```python
from build123d import *

# Parameters (mm, degrees)
SKETCH3_W               = 120
SKETCH3_H               = 85
BOSS_EXTRUDE1_DEPTH     = 5
SKETCH4_W               = 45
SKETCH4_H               = 18.75
BOSS_EXTRUDE2_DEPTH     = 20
SKETCH6_W               = 45
SKETCH6_H               = 2
BOSS_EXTRUDE3_DEPTH     = 40
CUT_EXTRUDE1_DEPTH      = 87.204698248
CUT_EXTRUDE1_DEPTH_BACK = 20
SKETCH7_W               = 4
SKETCH7_H               = 2
SKETCH8_W               = 10
SKETCH8_H               = 20
BOSS_EXTRUDE4_DEPTH     = 9
BOSS_EXTRUDE5_DEPTH     = 5.5
SKETCH10_W              = 2
SKETCH10_H              = 5.5
CUT_EXTRUDE2_DEPTH      = 91.627068942
SKETCH11_W              = 10
SKETCH11_H              = 10
BOSS_EXTRUDE6_DEPTH     = 2
SKETCH12_W              = 10
SKETCH12_H              = 10
BOSS_EXTRUDE7_DEPTH     = 9
SKETCH13_W              = 2.4
SKETCH13_H              = 10
BOSS_EXTRUDE8_DEPTH     = 4.5
SKETCH14_W              = 10
SKETCH14_H              = 5
BOSS_EXTRUDE9_DEPTH     = 2
SKETCH15_R              = 1.3
BOSS_EXTRUDE10_DEPTH    = 8
SKETCH16_W              = 9
SKETCH16_H              = 1.5
BOSS_EXTRUDE11_DEPTH    = 8
SKETCH18_W              = 120
SKETCH18_H              = 5
BOSS_EXTRUDE12_DEPTH    = 5
SKETCH19_W              = 90
SKETCH19_H              = 5
BOSS_EXTRUDE13_DEPTH    = 30
SKETCH17_W              = 55
SKETCH17_H              = 83
CUT_EXTRUDE3_DEPTH      = 2
SKETCH20_W              = 61
SKETCH20_H              = 90
SKETCH20_W_2            = 55
SKETCH20_H_2            = 83
BOSS_EXTRUDE14_DEPTH    = 6
SKETCH21_W              = 2
SKETCH21_H              = 90
CUT_EXTRUDE4_DEPTH      = 110.344638643
SKETCH22_W              = 5
SKETCH22_H              = 22.75
CUT_EXTRUDE5_DEPTH      = 16
SKETCH23_W              = 2
SKETCH23_H              = 20
BOSS_EXTRUDE15_DEPTH    = 11
FILLET1_R               = 10
FILLET2_R               = 10
SKETCH24_W              = 0.1
SKETCH24_H              = 5.5
CUT_EXTRUDE6_DEPTH      = 8
SKETCH25_W              = 5.2
SKETCH25_H              = 0.1
BOSS_EXTRUDE16_DEPTH    = 5


with BuildPart() as part:
    # Sketch3 → Boss-Extrude1 (new body)
    with BuildSketch(Plane(origin=(0, 0, 0), x_dir=(1, 0, 0), z_dir=(0, 1, 0))):
        Rectangle(SKETCH3_W, SKETCH3_H)
    extrude(amount=BOSS_EXTRUDE1_DEPTH)

    # Sketch4 → Boss-Extrude2 (add)
    with BuildSketch(Plane(origin=(0, 5, 0), x_dir=(1, 0, 0), z_dir=(0, 1, 0))):
        with Locations((37.5, 0)):
            Rectangle(SKETCH4_W, SKETCH4_H)
    extrude(amount=BOSS_EXTRUDE2_DEPTH)

    # Sketch6 → Boss-Extrude3 (add)
    with BuildSketch(Plane(origin=(0, 5, 0), x_dir=(1, 0, 0), z_dir=(0, 1, 0))):
        with Locations((37.5, 10.375)):
            Rectangle(SKETCH6_W, SKETCH6_H)
        with Locations((37.5, -10.375)):
            Rectangle(SKETCH6_W, SKETCH6_H)
    extrude(amount=BOSS_EXTRUDE3_DEPTH)

    # Sketch7 → Cut-Extrude1 (cut, two sides: drawn at the far end of the back side and taken through both)
    with BuildSketch(Plane(origin=(0, 45, 0), x_dir=(1, 0, 0), z_dir=(0, 1, 0)).offset(-CUT_EXTRUDE1_DEPTH_BACK)):
        with Locations((39, 10.375)):
            Rectangle(SKETCH7_W, SKETCH7_H)
    extrude(amount=CUT_EXTRUDE1_DEPTH + CUT_EXTRUDE1_DEPTH_BACK, mode=Mode.SUBTRACT)

    # Sketch8 → Boss-Extrude4 (add)
    with BuildSketch(Plane(origin=(0, 5, 0), x_dir=(1, 0, 0), z_dir=(0, 1, 0))):
        with Locations((-3, 1.625)):
            Rectangle(SKETCH8_W, SKETCH8_H)
    extrude(amount=BOSS_EXTRUDE4_DEPTH)

    # Sketch9 → Boss-Extrude5 (add)
    with BuildSketch(Plane(origin=(0, 14, 0), x_dir=(1, 0, 0), z_dir=(0, 1, 0))):
        Polygon((-8, -8.375), (2, -8.375), (2, 1.625), (-0.75, 1.625), (-0.75, -6.375), (-5.25, -6.375), (-5.25, 1.625), (-8, 1.625), align=None)
    extrude(amount=BOSS_EXTRUDE5_DEPTH)

    # Sketch10 → Cut-Extrude2 (cut, through all)
    with BuildSketch(Plane.XY.offset(8.375)):
        with Locations((-3, 16.75)):
            Rectangle(SKETCH10_W, SKETCH10_H)
    extrude(amount=-CUT_EXTRUDE2_DEPTH, mode=Mode.SUBTRACT)

    # Sketch11 → Boss-Extrude6 (add)
    with BuildSketch(Plane(origin=(0, 19.5, 0), x_dir=(1, 0, 0), z_dir=(0, 1, 0))):
        with Locations((-3, -3.375)):
            Rectangle(SKETCH11_W, SKETCH11_H)
    extrude(amount=BOSS_EXTRUDE6_DEPTH)

    # Sketch12 → Boss-Extrude7 (add)
    with BuildSketch(Plane(origin=(0, 5, 0), x_dir=(1, 0, 0), z_dir=(0, 1, 0))):
        with Locations((-3, -26.375)):
            Rectangle(SKETCH12_W, SKETCH12_H)
    extrude(amount=BOSS_EXTRUDE7_DEPTH)

    # Sketch13 → Boss-Extrude8 (add)
    with BuildSketch(Plane(origin=(0, 14, 0), x_dir=(1, 0, 0), z_dir=(0, 1, 0))):
        with Locations((-6.8, -26.375)):
            Rectangle(SKETCH13_W, SKETCH13_H)
        with Locations((0.8, -26.375)):
            Rectangle(SKETCH13_W, SKETCH13_H)
    extrude(amount=BOSS_EXTRUDE8_DEPTH)

    # Sketch14 → Boss-Extrude9 (add)
    with BuildSketch(Plane(origin=(0, 18.5, 0), x_dir=(1, 0, 0), z_dir=(0, 1, 0))):
        with Locations((-3, -23.875)):
            Rectangle(SKETCH14_W, SKETCH14_H)
    extrude(amount=BOSS_EXTRUDE9_DEPTH)

    # Sketch15 → Boss-Extrude10 (add)
    with BuildSketch(Plane(origin=(0, 5, 0), x_dir=(1, 0, 0), z_dir=(0, 1, 0))):
        with Locations(Location((33.5, 37.5, 0), (0, 0, 90))):
            Circle(SKETCH15_R)
        with Locations(Location((53.5, 37.5, 0), (0, 0, 90))):
            Circle(SKETCH15_R)
        with Locations(Location((53.5, 17.5, 0), (0, 0, 90))):
            Circle(SKETCH15_R)
        with Locations(Location((33.5, 17.5, 0), (0, 0, 90))):
            Circle(SKETCH15_R)
    extrude(amount=BOSS_EXTRUDE10_DEPTH)

    # Sketch16 → Boss-Extrude11 (add)
    with BuildSketch(Plane(origin=(0, 5, 0), x_dir=(1, 0, 0), z_dir=(0, 1, 0))):
        with Locations((55.5, -12.125)):
            Rectangle(SKETCH16_W, SKETCH16_H)
        Polygon((51, -25.375), (32, -25.375), (32, -27.375), (60, -27.375), (60, -25.375), align=None)
        with Locations((55.5, -24.625)):
            Rectangle(SKETCH16_W, SKETCH16_H)
    extrude(amount=BOSS_EXTRUDE11_DEPTH)

    # Sketch18 → Boss-Extrude12 (add)
    with BuildSketch(Plane.XY.offset(42.5)):
        with Locations((0, 2.5)):
            Rectangle(SKETCH18_W, SKETCH18_H)
    extrude(amount=BOSS_EXTRUDE12_DEPTH)

    # Sketch19 → Boss-Extrude13 (add)
    with BuildSketch(Plane.ZY.offset(60)):
        with Locations((2.5, 2.5)):
            Rectangle(SKETCH19_W, SKETCH19_H)
    extrude(amount=BOSS_EXTRUDE13_DEPTH)

    # Sketch17 → Cut-Extrude3 (cut)
    with BuildSketch(Plane(origin=(0, 5, 0), x_dir=(1, 0, 0), z_dir=(0, 1, 0))):
        with Locations((-57.5, -2)):
            Rectangle(SKETCH17_W, SKETCH17_H)
    extrude(amount=-CUT_EXTRUDE3_DEPTH, mode=Mode.SUBTRACT)

    # Sketch20 → Boss-Extrude14 (add)
    with BuildSketch(Plane(origin=(0, 5, 0), x_dir=(1, 0, 0), z_dir=(0, 1, 0))):
        with Locations((-57.5, -2.5)):
            Rectangle(SKETCH20_W, SKETCH20_H)
        with Locations((-57.5, -2)):
            Rectangle(SKETCH20_W_2, SKETCH20_H_2, mode=Mode.SUBTRACT)
    extrude(amount=BOSS_EXTRUDE14_DEPTH)

    # Sketch21 → Cut-Extrude4 (cut, through all)
    with BuildSketch(Plane(origin=(0, 5, 0), x_dir=(1, 0, 0), z_dir=(0, 1, 0))):
        with Locations((-89, -2.5)):
            Rectangle(SKETCH21_W, SKETCH21_H)
    extrude(amount=-CUT_EXTRUDE4_DEPTH, mode=Mode.SUBTRACT)

    # Sketch22 → Cut-Extrude5 (cut)
    with BuildSketch(Plane(origin=(0, 45, 0), x_dir=(1, 0, 0), z_dir=(0, 1, 0))):
        with Locations((30, 0)):
            Rectangle(SKETCH22_W, SKETCH22_H)
    extrude(amount=-CUT_EXTRUDE5_DEPTH, mode=Mode.SUBTRACT)

    # Sketch23 → Boss-Extrude15 (add)
    with BuildSketch(Plane.ZY.offset(-15)):
        with Locations((-10.375, 35)):
            Rectangle(SKETCH23_W, SKETCH23_H)
        with Locations((10.375, 35)):
            Rectangle(SKETCH23_W, SKETCH23_H)
    extrude(amount=BOSS_EXTRUDE15_DEPTH)

    # Fillet1
    fillet1_edges = [part.edges().sort_by_distance(p)[0] for p in [
        (15, 25, -10.375),
        (15, 25, 10.375),
    ]]
    fillet(fillet1_edges, radius=FILLET1_R)

    # Fillet2
    fillet2_edges = [part.edges().sort_by_distance(p)[0] for p in [
        (4, 25, -10.375),
        (4, 25, 10.375),
    ]]
    fillet(fillet2_edges, radius=FILLET2_R)

    # Sketch24 → Cut-Extrude6 (cut)
    with BuildSketch(Plane(origin=(0, 0, -1.625), x_dir=(-1, 0, 0), z_dir=(0, 0, -1))):
        Polygon((0.75, 19.5), (5.25, 19.5), (5.35, 19.5), (5.35, 19.6), (0.65, 19.6), (0.65, 19.5), align=None)
        with Locations((5.3, 16.75)):
            Rectangle(SKETCH24_W, SKETCH24_H)
        with Locations((0.7, 16.75)):
            Rectangle(SKETCH24_W, SKETCH24_H)
    extrude(amount=-CUT_EXTRUDE6_DEPTH, mode=Mode.SUBTRACT)

    # Sketch25 → Boss-Extrude16 (add)
    with BuildSketch(Plane(origin=(0, 0, 21.375), x_dir=(-1, 0, 0), z_dir=(0, 0, -1))):
        with Locations((3, 18.45)):
            Rectangle(SKETCH25_W, SKETCH25_H)
    extrude(amount=-BOSS_EXTRUDE16_DEPTH)


solid = part.part
```
Can you work these out from the model? Positions are in its coordinate system, mm. A direction names the side the tool comes from. Round coordinates to 2 decimals unless told otherwise and drop trailing zeros. Loops run counter-clockwise (first coordinate to the right, second up) from the corner with the lowest first, then second, coordinate; pieces in that order, holes last. Notation, with made-up numbers: M 80.25,49.5 L 114.25,49.5 A26 cw 114.25,68.5 Z; hole C 82,-32.5 d2. An arc over 180 degrees is marked long. Answer as a JSON object with one key per item and string values. Group by question number.
Q1. Imagine slicing it at C-C, the plane z = 29.5. Please give me the cut outline in (x, y), then the cut area to 3 significant figures.
Q2. Imagine slicing it at A-A, the plane y = 41.5. Please give me the cut outline in (x, z) (3 decimals).
Q3. Imagine slicing it at B-B, the plane x = -69. Please give me the cut outline in (y, z).
Q4. On a 3-axis mill with a long thin cutter (end or side, diameter ignored), from which of +Z, -Z, +X, -X, +Y, -Y can I reach the whole of each face in a straight line? I mean faces 1 (the flat face through (-8, 11, 1)), 2 (the cylindrical face through (13.555, 20.178, -10.361)), 3 (the flat face through (-0.65, 17, 2)), 4 (the flat face through (49, 13, 26)), 5 (the flat face through (-3, 21.5, 3)). Say none if no direction works.
Q5. We'd pull the mould along X, two halves only. Please class faces 6 (the flat face through (-3, 14, -4)), 7 (the flat face through (-3, 10, 31.375)), 8 (the cylindrical face through (13.555, 20.178, 10.389)): +X half, -X half, draft (parallel to the pull), parting line (faces both ways), or undercut.
Q6. Will these pins go through, and if not, where does the flat tip stop? pin 1 (0.8 mm diameter, centred on x = 54.5, z = 12.5, fed in from +Y); pin 2 (4 mm diameter, centred on x = 54, y = 9.5, fed in from -Z); pin 3 (2 mm diameter, centred on x = -68.5, z = 2, fed in from +Y).
Q7. Imagine slicing it at D-D, the plane z = -25.5. Please give me the cut outline in (x, y).
Q8. Please list where these lines run through material, in increasing order: L1, parallel to X at y = 8, z = -7; L2, parallel to Z at x = 25, y = 33 (3 decimals); L3, parallel to X at y = 9.5, z = -16.5.
Findings:
{
 "1": {"outline": "M -88,0 L 60,0 L 60,5 L 2,5 L 2,18.5 L -0.4,18.5 L -0.4,14 L -5.6,14 L -5.6,18.5 L -8,18.5 L -8,5 L -27,5 L -27,11 L -30,11 L -30,3 L -85,3 L -85,11 L -88,11 Z", "area": "778 mm2"},
 "2": {"outline": "M 4,-11.375 L 27.5,-11.375 L 27.5,-9.375 L 4,-9.375 Z; M 4,9.375 L 27.5,9.375 L 27.5,11.375 L 4,11.375 Z; M 32.5,-11.375 L 37,-11.375 L 37,-9.375 L 32.5,-9.375 Z; M 32.5,9.375 L 60,9.375 L 60,11.375 L 32.5,11.375 Z; M 41,-11.375 L 60,-11.375 L 60,-9.375 L 41,-9.375 Z"},
 "3": {"outline": "M 0,-42.5 L 11,-42.5 L 11,-39.5 L 3,-39.5 L 3,43.5 L 11,43.5 L 11,47.5 L 0,47.5 Z"},
 "4": {"face 1": "+Z, -Z, +Y", "face 2": "+Z, -Z, -X", "face 3": "-Z", "face 4": "+Z, +X, +Y", "face 5": "+Z, -Z, -X, +Y"},
 "5": {"face 6": "undercut", "face 7": "draft", "face 8": "-X half"},
 "6": {"pin 1": "stops at y = 13", "pin 2": "stops at z = -38.8", "pin 3": "stops at y = 3"},
 "7": {"outline": "M -88,0 L 60,0 L 60,5 L -27,5 L -27,11 L -30,11 L -30,3 L -85,3 L -85,11 L -88,11 Z"},
 "8": {"L1": "x = -88 to -85, -30 to -27, -8 to 2, 15 to 60", "L2": "z = -11.375 to -9.375, 9.375 to 11.375", "L3": "x = -88 to -85, -30 to -27, 32.67 to 34.33, 52.67 to 54.33"}
}
